Part model, mm, in its own coordinate system. Face numbers are marked on the shaded views. A direction names the side the tool comes from. Give positions to 0.01 mm unless a question says otherwise; leave off trailing zeros. Loops run counter-clockwise (first coordinate to the right, second up) from the corner with the lowest first, then second, coordinate; pieces in that order, holes last. Notation, with made-up numbers: M 29.25,-19.5 L 64.25,-19.5 A31 ccw 64.25,14.5 Z; hole C -28.75,47.25 d2. An arc over 180 degrees is marked long. Answer in a Markdown table with one row per item.
from build123d import *

# Parameters (mm, degrees)
ESQUISSE1_W             = 34
ESQUISSE1_H             = 100
BOSS_EXTRU_1_DEPTH      = 18
COQUE1_T                = 2
ESQUISSE2_W             = 34
ESQUISSE2_H             = 18
ENL_V_MAT_EXTRU_1_DEPTH = 18
CONG_1_R                = 2
ESQUISSE5_W             = 1.999683034
ESQUISSE5_H             = 104
BOSS_EXTRU_2_DEPTH      = 3
ESQUISSE6_W             = 1.999683034
ESQUISSE6_H             = 104
BOSS_EXTRU_3_DEPTH      = 3
ESQUISSE7_W             = 44
ESQUISSE7_H             = 1.999683034
BOSS_EXTRU_4_DEPTH      = 4
CONG_2_R                = 4
CONG_3_R                = 2
CONG_5_R                = 2
ESQUISSE8_R             = 1.5
ENL_V_MAT_EXTRU_2_DEPTH = 10


with BuildPart() as part:
    # Esquisse1 → Boss.-Extru.1 (new body)
    with BuildSketch(Plane.XY):
        with Locations((17, 50)):
            Rectangle(ESQUISSE1_W, ESQUISSE1_H)
    extrude(amount=BOSS_EXTRU_1_DEPTH)

    # Coque1
    coque1_openings = [part.faces().sort_by_distance(p)[0] for p in [
        (17, 50, 0),
    ]]
    offset(amount=COQUE1_T, openings=coque1_openings, kind=Kind.INTERSECTION)

    # Esquisse2 → Enlèv. mat.-Extru.1 (cut)
    with BuildSketch(Plane.XZ.offset(-100)):
        with Locations((17, 9)):
            Rectangle(ESQUISSE2_W, ESQUISSE2_H)
    extrude(amount=-ENL_V_MAT_EXTRU_1_DEPTH, mode=Mode.SUBTRACT)

    # Congé1
    cong_1_edges = [part.edges().sort_by_distance(p)[0] for p in [
        (36, 50, 20),
        (-2, 50, 20),
        (17, -2, 20),
    ]]
    fillet(cong_1_edges, radius=CONG_1_R)

    # Esquisse5 → Boss.-Extru.2 (add)
    with BuildSketch(Plane.ZY.offset(2)):
        with Locations((0.999841517, 50)):
            Rectangle(ESQUISSE5_W, ESQUISSE5_H)
    extrude(amount=BOSS_EXTRU_2_DEPTH)

    # Esquisse6 → Boss.-Extru.3 (add)
    with BuildSketch(Plane(origin=(36, 0, 0), x_dir=(0, 0, -1), z_dir=(1, 0, 0))):
        with Locations((-0.999841517, 50)):
            Rectangle(ESQUISSE6_W, ESQUISSE6_H)
    extrude(amount=BOSS_EXTRU_3_DEPTH)

    # Esquisse7 → Boss.-Extru.4 (add)
    with BuildSketch(Plane.XZ.offset(2)):
        with Locations((17, 0.999841517)):
            Rectangle(ESQUISSE7_W, ESQUISSE7_H)
    extrude(amount=BOSS_EXTRU_4_DEPTH)

    # Congé2
    # the kernel refuses this fillet: 4 mm, written as the material it takes off along each edge
    with BuildSketch(Plane(origin=(2, 2, 20), x_dir=(-1, 0, 0), z_dir=(0, 1, 0))) as cong_2_piece_1:
        with BuildLine():
            CenterArc((2, -2), 2, 0, 90)
            Line((4, -2), (4, 0))
            Line((4, 0), (2, 0))
        make_face()
    revolve(axis=Axis((2, 2, 20), (0, 0, 1)), revolution_arc=90, mode=Mode.SUBTRACT)
    with BuildSketch(Plane(origin=(32, 2, 20), x_dir=(0, -1, 0), z_dir=(-1, 0, 0))) as cong_2_piece_2:
        with BuildLine():
            CenterArc((2, -2), 2, 0, 90)
            Line((4, -2), (4, 0))
            Line((4, 0), (2, 0))
        make_face()
    revolve(axis=Axis((32, 2, 20), (0, 0, 1)), revolution_arc=90, mode=Mode.SUBTRACT)
    with BuildSketch(Plane(origin=(36, -2, 1.999683034), x_dir=(-1, 0, 0), z_dir=(0, 0, 1)), Plane(origin=(-2, -2, 20), x_dir=(1, 0, 0), z_dir=(0, 0, -1))) as cong_2_piece_3:
        with BuildLine():
            CenterArc((CONG_2_R, -CONG_2_R), CONG_2_R, 90, 90)
            Line((0, -CONG_2_R), (0, 0))
            Line((0, 0), (CONG_2_R, 0))
        make_face()
    extrude(amount=18.000316966, mode=Mode.SUBTRACT)
    with BuildSketch(Plane(origin=(39, -6, 11.999683034), x_dir=(0, 1, 0), z_dir=(0, 0, -1))) as cong_2_piece_4:
        with BuildLine():
            CenterArc((CONG_2_R, -CONG_2_R), CONG_2_R, 90, 90)
            Line((0, -CONG_2_R), (0, 0))
            Line((0, 0), (CONG_2_R, 0))
        make_face()
    extrude(amount=21.999683034, mode=Mode.SUBTRACT)
    with BuildSketch(Plane(origin=(-5, -6, -10), x_dir=(1, 0, 0), z_dir=(0, 0, 1))) as cong_2_piece_5:
        with BuildLine():
            CenterArc((CONG_2_R, CONG_2_R), CONG_2_R, 180, 90)
            Line((0, CONG_2_R), (0, 0))
            Line((0, 0), (CONG_2_R, 0))
        make_face()
    extrude(amount=21.999683034, mode=Mode.SUBTRACT)

    # Congé3
    cong_3_edges = [part.edges().sort_by_distance(p)[0] for p in [
        (17, -2, 1.999683034),
        (-2, 52, 1.999683034),
        (34.828427125, -0.828427125, 1.999683034),
        (-0.828427125, -0.828427125, 1.999683034),
        (36, 52, 1.999683034),
    ]]
    fillet(cong_3_edges, radius=CONG_3_R)

    # Congé5
    cong_5_edges = [part.edges().sort_by_distance(p)[0] for p in [
        (0, 51, 0),
        (17, 0, 0),
        (34, 51, 0),
    ]]
    fillet(cong_5_edges, radius=CONG_5_R)

    # Esquisse8 → Enlèv. mat.-Extru.2 (cut)
    with BuildSketch(Plane.XY.offset(20)):
        with Locations((17, 76)):
            Circle(ESQUISSE8_R)
    extrude(amount=-ENL_V_MAT_EXTRU_2_DEPTH, mode=Mode.SUBTRACT)


solid = part.part
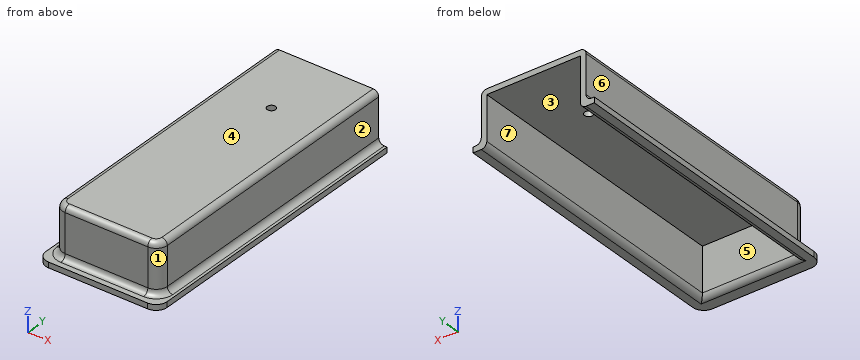
(1) Which spindle directions (+Z, -Z, +X, -X, +Y, -Y) get a long thin tool onto all of the face, cutting with end or side? Do the marked faces 1, 2 and 3. Say none if no direction does.
Recorded:
| item | result |
|---|---|
| face 1 | +Z, +X, -Y |
| face 2 | +Z, +X, +Y, -Y |
| face 3 | -Z, +Y |
(2) Pull direction X, two halves, no side cores. Call the marked faces 4, 5, 6 and 7: +X half, -X half, draft (parallel to the pull), parting line (faces both ways), or undercut.
Recorded:
| item | result |
|---|---|
| face 4 | draft |
| face 5 | undercut |
| face 6 | -X half |
| face 7 | undercut |
(3) Saw through at B-B (y = 76). Write the cut outline in (x, z).
Recorded:
| item | result |
|---|---|
| outline | M -5,0 L -2,0 A2 ccw 0,2 L 0,18 L 15.5,18 L 15.5,20 L 0,20 A2 ccw -2,18 L -2,4 A2 cw -4,2 L -5,2 Z; M 18.5,18 L 34,18 L 34,2 A2 ccw 36,0 L 39,0 L 39,2 L 38,2 A2 cw 36,4 L 36,18 A2 ccw 34,20 L 18.5,20 Z |
(4) Saw through at C-C (x = 3.5). Write the cut outline in (y, z).
Recorded:
| item | result |
|---|---|
| outline | M -6,0 L -2,0 A2 ccw 0,2 L 0,18 L 102,18 L 102,20 L 0,20 A2 ccw -2,18 L -2,4 A2 cw -4,2 L -6,2 Z |
(5) Pin check, flat tips, straight feed: pin 1 Ø5 at (x, z) = (12, 4.5) entering from +Y; pin 2 Ø4 at (y, z) = (28, 13.5) entering from +X; pin 3 Ø5 at (x, y) = (3.5, 49.5) entering from -Z. Stop position of each tip, or through.
Recorded:
| item | result |
|---|---|
| pin 1 | stops at y = 0 |
| pin 2 | stops at x = 36 |
| pin 3 | stops at z = 18 |
(6) Saw through at A-A (x = 17). Write the cut outline in (y, z), plus the area to 3 significant figures.
Recorded:
| item | result |
|---|---|
| outline | M -6,0 L -2,0 A2 ccw 0,2 L 0,18 L 74.5,18 L 74.5,20 L 0,20 A2 ccw -2,18 L -2,4 A2 cw -4,2 L -6,2 Z; M 77.5,18 L 102,18 L 102,20 L 77.5,20 Z |
| area | 245 mm^2 |
(7) Saw through at D-D (y = 44.5). Write the cut outline in (x, z).
Recorded:
| item | result |
|---|---|
| outline | M -5,0 L -2,0 A2 ccw 0,2 L 0,18 L 34,18 L 34,2 A2 ccw 36,0 L 39,0 L 39,2 L 38,2 A2 cw 36,4 L 36,18 A2 ccw 34,20 L 0,20 A2 ccw -2,18 L -2,4 A2 cw -4,2 L -5,2 Z |
(8) Drill centre lines: line 1 along X through (y, z) = (63.5, 17.5); line 2 along Z through (x, y) = (12.5, 38); line 3 along Y through (x, z) = (23, 12.75). Where is each one in solid material? Low to high.
Recorded:
| item | result |
|---|---|
| line 1 | x = -2 to 0, 34 to 36 |
| line 2 | z = 18 to 20 |
| line 3 | y = -2 to 0 |
